```python
from build123d import *

# Parameters (mm, degrees)
SKETCH1_W           = 30
SKETCH1_H           = 44
BOSS_EXTRUDE1_DEPTH = 3
CUT_EXTRUDE1_DEPTH  = 27.795522014
SKETCH3_W           = 15
SKETCH3_H           = 3
SKETCH3_W_2         = 3
SKETCH3_H_2         = 15
BOSS_EXTRUDE2_DEPTH = 3
FILLET1_R           = 20


with BuildPart() as part:
    # Sketch1 → Boss-Extrude1 (new body)
    with BuildSketch(Plane(origin=(0, 0, 0), x_dir=(1, 0, 0), z_dir=(0, 1, 0))):
        Rectangle(SKETCH1_W, SKETCH1_H)
    extrude(amount=BOSS_EXTRUDE1_DEPTH)

    # Sketch2 → Cut-Extrude1 (cut, through all)
    with BuildSketch(Plane(origin=(0, 3, 0), x_dir=(1, 0, 0), z_dir=(0, 1, 0))):
        with BuildLine():
            Line((-15, -7), (-15, 22))
            Line((-15, 22), (0, 22))
            ThreePointArc((0, 22), (-11.028000253, 9.324827717), (-15, -7))
        make_face()
    extrude(amount=-CUT_EXTRUDE1_DEPTH, mode=Mode.SUBTRACT)

    # Sketch3 → Boss-Extrude2 (add)
    with BuildSketch(Plane(origin=(0, 3, 0), x_dir=(1, 0, 0), z_dir=(0, 1, 0))):
        with Locations((0, -23.5)):
            Rectangle(SKETCH3_W, SKETCH3_H)
        with Locations((16.5, 0)):
            Rectangle(SKETCH3_W_2, SKETCH3_H_2)
    extrude(amount=-BOSS_EXTRUDE2_DEPTH)

    # Fillet1
    fillet1_edges = [part.edges().sort_by_distance(p)[0] for p in [
        (0, 1.5, -22),
    ]]
    fillet(fillet1_edges, radius=FILLET1_R)


solid = part.part
```
Check sheet for the modelled part. Datum: model origin and axes. Units: mm. A direction names the side the tool comes from. Round coordinates to 2 decimals unless told otherwise and drop trailing zeros. Loops run counter-clockwise (first coordinate to the right, second up) from the corner with the lowest first, then second, coordinate; pieces in that order, holes last. Notation, with made-up numbers: (11, 4) - (24, 4) arc R8 cw to (24, 13) - close; hole circle Ø11 at (22, 20.5). An arc over 180 degrees is marked (long way). Answer as a JSON object with one key per item and string values. Group by question number.
Q1. Sectioned sample at C-C, the plane x = 10.5. Enter the section's corners in (y, z), plus the area to 3 significant figures.
Q2. Gauge pin test, flat ends, axial feed: P1, Ø0.9, axis at y = 1.5, z = 16, coming from the +X side; P2, Ø1.5, axis at x = -11, y = 1, coming from the +Z side; P3, Ø0.9, axis at x = 16, y = 1.5, coming from the -Z side. Record the tip position at first contact, or that the pin passes through.
Q3. Sectioned sample at A-A, the plane y = 2.15. Enter the section's corners in (x, z), plus the area to 3 significant figures.
Q4. Sectioned sample at B-B, the plane z = 22.5. Enter the section's corners in (x, y).
Q5. Scan lines: line 1 along Z through (x, y) = (14.5, 1.85); line 2 along X through (y, z) = (1.4, 14.5); line 3 along X through (y, z) = (1.6, -15). Record each from-to range of solid material in increasing order. Write a range as [from, to].
Q6. Set-up check for faces 1 (the face through (15, 1, -15)), 2 (the face through (-7.5, 2, 24)), 3 (the face through (16, 2, 7.5)): record each of +Z, -Z, +X, -X, +Y, -Y from which the full face is reachable in a straight line by a thin tool's end or side.
Solution:
{
 "1": {"outline": "(0, -22) - (3, -22) - (3, 22) - (0, 22) - close", "area": "132 mm²"},
 "2": {"P1": "stops at x = 15", "P2": "stops at z = 22", "P3": "stops at z = -7.5"},
 "3": {"outline": "(-15, 7) arc R35.53 ccw to (-8.43, -13.59) arc R20 ccw to (7.87, -22) - (15, -22) - (15, -7.5) - (18, -7.5) - (18, 7.5) - (15, 7.5) - (15, 22) - (7.5, 22) - (7.5, 25) - (-7.5, 25) - (-7.5, 22) - (-15, 22) - close", "area": "1,270 mm²"},
 "4": {"outline": "(-7.5, 0) - (7.5, 0) - (7.5, 3) - (-7.5, 3) - close"},
 "5": {"line 1": "z = [-22, 22]", "line 2": "x = [-15, 15]", "line 3": "x = [-7.33, 15]"},
 "6": {"face 1": "-Z, +X, +Y, -Y", "face 2": "+Z, -X, +Y, -Y", "face 3": "+Z, +X, +Y, -Y"}
}
